Check sheet for the modelled part. Datum: model origin and axes. Units: mm. Give positions to 0.01 mm unless a question says otherwise; leave off trailing zeros. Write each loop counter-clockwise with the first axis right and the second up, starting at its lowest first coordinate (ties: lowest second). Pieces come first, ordered by that corner, then holes. Notation, with made-up numbers: M -35,81.5 L -22,81.5 A16 cw -22,91.5 Z; hole C 76.5,88.25 d11. An arc over 180 degrees is marked long. Write each question's results on one line, items separated by ' | '. Start each with the question number.
from build123d import *

# Parameters (mm, degrees)
SKETCH2_R           = 7.5
BOSS_EXTRUDE1_DEPTH = 100
CUT_EXTRUDE1_DEPTH  = 50
SKETCH5_R           = 2.5
CUT_EXTRUDE2_DEPTH  = 10
SKETCH6_R           = 2.5
CUT_EXTRUDE3_DEPTH  = 7


with BuildPart() as part:
    # Sketch2 → Boss-Extrude1 (new body)
    with BuildSketch(Plane.XY):
        Circle(SKETCH2_R)
    extrude(amount=BOSS_EXTRUDE1_DEPTH)

    # Sketch3 → Cut-Extrude1 (cut, symmetric)
    with BuildSketch(Plane(origin=(0, 0, 0), x_dir=(1, 0, 0), z_dir=(0, 1, 0))):
        Polygon((7.5, 0), (-16.600154846, -13.914230888), (-16.600154846, 6.795957579), (7.5, 6.795957579), align=None)
        Polygon((7.5, -100), (-10.5, -68.823085464), (-10.5, -108.823085464), (7.5, -108.823085464), align=None)
    extrude(amount=CUT_EXTRUDE1_DEPTH, both=True, mode=Mode.SUBTRACT)

    # Sketch5 → Cut-Extrude2 (cut)
    with BuildSketch(Plane(origin=(1.875, 0, 3.247595264), x_dir=(-0.8660254037844379, 0, 0.5000000000000013), z_dir=(-0.5000000000000013, 0, -0.8660254037844379))):
        with Locations((4.825317547, 0)):
            Circle(SKETCH5_R)
    extrude(amount=-CUT_EXTRUDE2_DEPTH, mode=Mode.SUBTRACT)

    # Sketch6 → Cut-Extrude3 (cut)
    with BuildSketch(Plane(origin=(-37.676270189, 0, 21.752404736), x_dir=(0.5000000000000042, 0, 0.8660254037844363), z_dir=(-0.8660254037844363, 0, 0.5000000000000042))):
        with Locations((68.352540378, 0)):
            Circle(SKETCH6_R)
    extrude(amount=-CUT_EXTRUDE3_DEPTH, mode=Mode.SUBTRACT)


solid = part.part
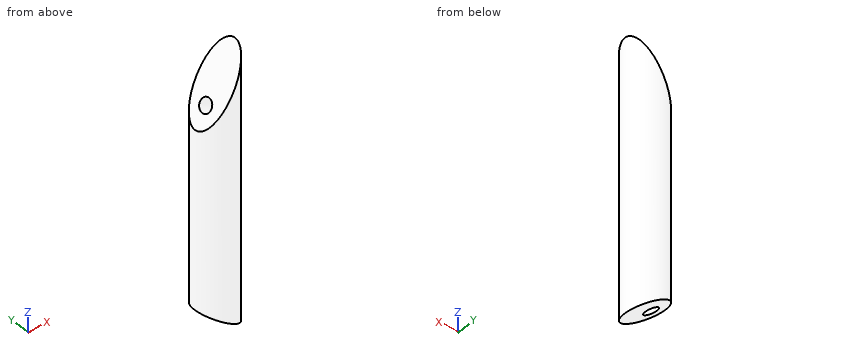
Q1. Depth check by flat-ended pin: pin 1 Ø3 at (y, z) = (-6, 49.5) entering from -X; pin 2 Ø1 at (y, z) = (-2, 71) entering from -X; pin 3 Ø5 at (y, z) = (-4.5, 77) entering from -X. Enter the tip coordinate at first touch or a pass-through.
Q2. Section check B-B on y = -1.5. Record the boundary of the cut face in (x, z), plus the area to 3 significant figures.
Q3. Section check A-A on z = 48.5. Record the boundary of the cut face in (x, y), plus the area to 3 significant figures.
Q4. Section check D-D on x = -5.75. Record the boundary of the cut face in (y, z), plus the area to 3 significant figures.
Q5. Scan lines: L1, parallel to Z at x = 1.25, y = 0.5; L2, parallel to Z at x = 1, y = -0.25; L3, parallel to Y at x = 5.5, z = 88. Record each from-to range of solid material in increasing order.
Q6. Section check C-C on x = 6. Record the boundary of the cut face in (y, z), plus the area to 3 significant figures.
Check result:
1) pin 1: x = -6 | pin 2: x = -7.35 | pin 3: x = -6.9
2) outline: M -7.35,8.57 L -4.04,6.66 L 0.96,15.32 L 4.43,13.32 L -0.57,4.66 L 7.35,0.09 L 7.35,99.74 L -2.5,82.68 L 3.56,79.18 L 1.56,75.72 L -4.5,79.22 L -7.35,74.28 Z | area: 1,150 mm^2
3) outline: C 0,0 d15 | area: 177 mm^2
4) outline: M -4.82,7.65 L 4.82,7.65 L 4.82,77.05 L -4.82,77.05 Z | area: 668 mm^2
5) L1: 3.61 to 6.92, 15.16 to 75.38, 81.03 to 89.17 | L2: 3.75 to 6.41, 15.3 to 75.48, 81.22 to 88.74 | L3: -5.1 to 5.1
6) outline: M -4.5,0.87 L 4.5,0.87 L 4.5,97.4 L -4.5,97.4 Z | area: 869 mm^2
